The drawing under review shows one solid part. Ordinate dimensions are in mm from its lowest x, y, z. A direction names the side the tool comes from. Coordinates: 2 decimals unless noted, no trailing zeros. Write each loop counter-clockwise with the first axis right and the second up, starting at its lowest first coordinate (ties: lowest second). Pieces come first, ordered by that corner, then holes.
Q1. For probe 1 along X at (y, z) = (14.25, 15.25); probe 2 along Z at (x, y) = (16.25, 14.5); probe 3 along Y at (x, z) = (17.5, 19), list the stretches that pass through material, from the lowest coordinate up.
Q2. Insertion check: pin 1 (1.2 mm diameter, centred on x = 16.5, y = 13, fed in from -Z); pin 2 (0.9 mm diameter, centred on y = 14, z = 16.5, fed in from +X); pin 3 (1.2 mm diameter, centred on x = 4, y = 13.5, fed in from +Z); pin 4 (3 mm diameter, centred on x = 2, z = 18, fed in from -Y). Each pin has a flat end and moves straight along its axis. Give the tip position at first contact, or say it passes through.
Q3. Mouldability with a two-part tool opening along X and no side actions: class the marked faces 4, 5 and 6 as pulls with the +X half, pulls with the -X half, needs draft (parallel to the pull), parting line crosses it, or undercut.
Q4. Take a section at B-B (z = 20.25). Give the boundary of the cut face in (x, y), and give its area (3 significant figures).
Q5. Take a section at A-A (y = 13). Give the boundary of the cut face in (x, z).
Q6. Machinability: for the marked faces 1, 2 and 3, which of the approach directions +Z, -Z, +X, -X, +Y, -Y give a long, thin tool a straight path to every point of the face, cutting with its end or side? Answer none if there is none.
Q7. Take a section at C-C (x = 4). Give the boundary of the cut face in (y, z), and give its area (3 significant figures).
Q8. Take a section at D-D (y = 3). Give the boundary of the cut face in (x, z), and give its area (3 significant figures).
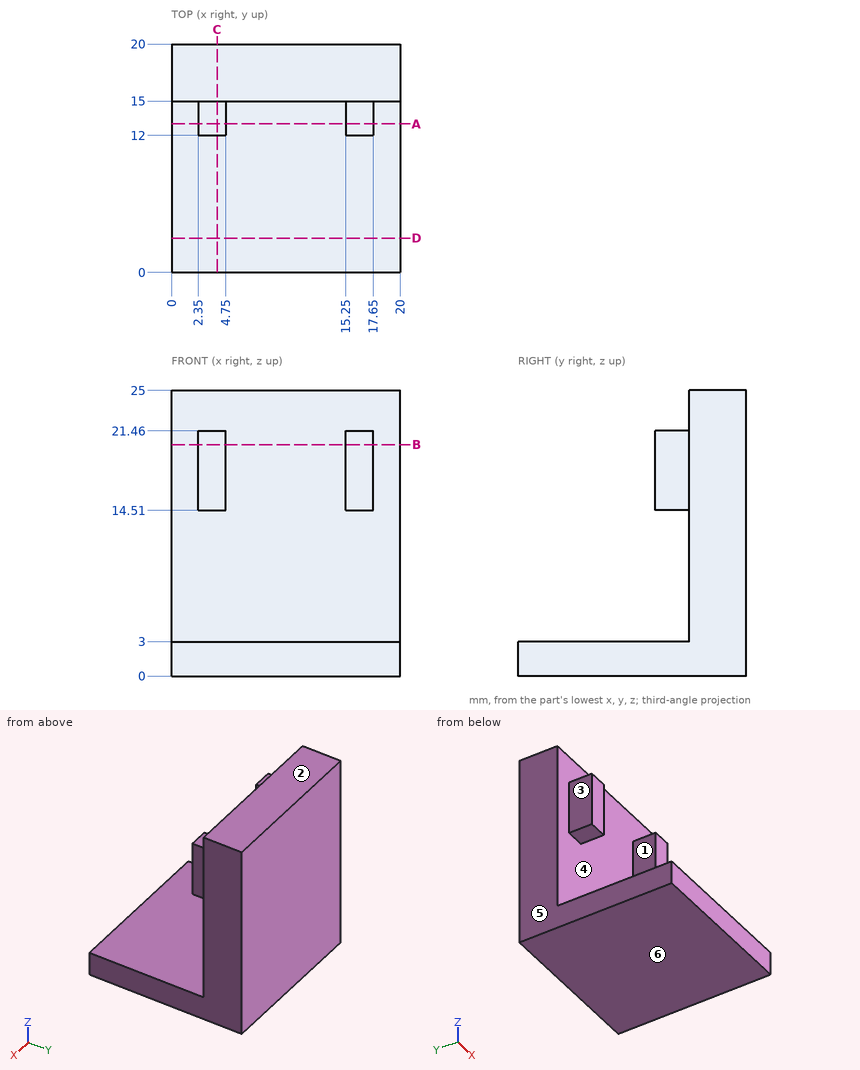
Response:
1. probe 1: x = 2.35 to 4.75, 15.25 to 17.65
1. probe 2: z = 0 to 3, 14.51 to 21.46
1. probe 3: y = 12 to 20
2. pin 1: stops at z = 0
2. pin 2: stops at x = 17.65
2. pin 3: stops at z = 21.46
2. pin 4: stops at y = 12
3. face 4: undercut
3. face 5: pulls with the -X half
3. face 6: needs draft
4. outline: (0, 15) - (2.35, 15) - (2.35, 12) - (4.75, 12) - (4.75, 15) - (15.25, 15) - (15.25, 12) - (17.65, 12) - (17.65, 15) - (20, 15) - (20, 20) - (0, 20) - close
4. area: 114 mm2
5. outline: (0, 0) - (20, 0) - (20, 3) - (0, 3) - close; (2.35, 14.51) - (4.75, 14.51) - (4.75, 21.46) - (2.35, 21.46) - close; (15.25, 14.51) - (17.65, 14.51) - (17.65, 21.46) - (15.25, 21.46) - close
6. face 1: +Z, -Y
6. face 2: +Z, +X, -X, +Y, -Y
6. face 3: +Z, -X, -Y
7. outline: (0, 0) - (20, 0) - (20, 25) - (15, 25) - (15, 21.46) - (12, 21.46) - (12, 14.51) - (15, 14.51) - (15, 3) - (0, 3) - close
7. area: 191 mm2
8. outline: (0, 0) - (20, 0) - (20, 3) - (0, 3) - close
8. area: 60.0 mm2
